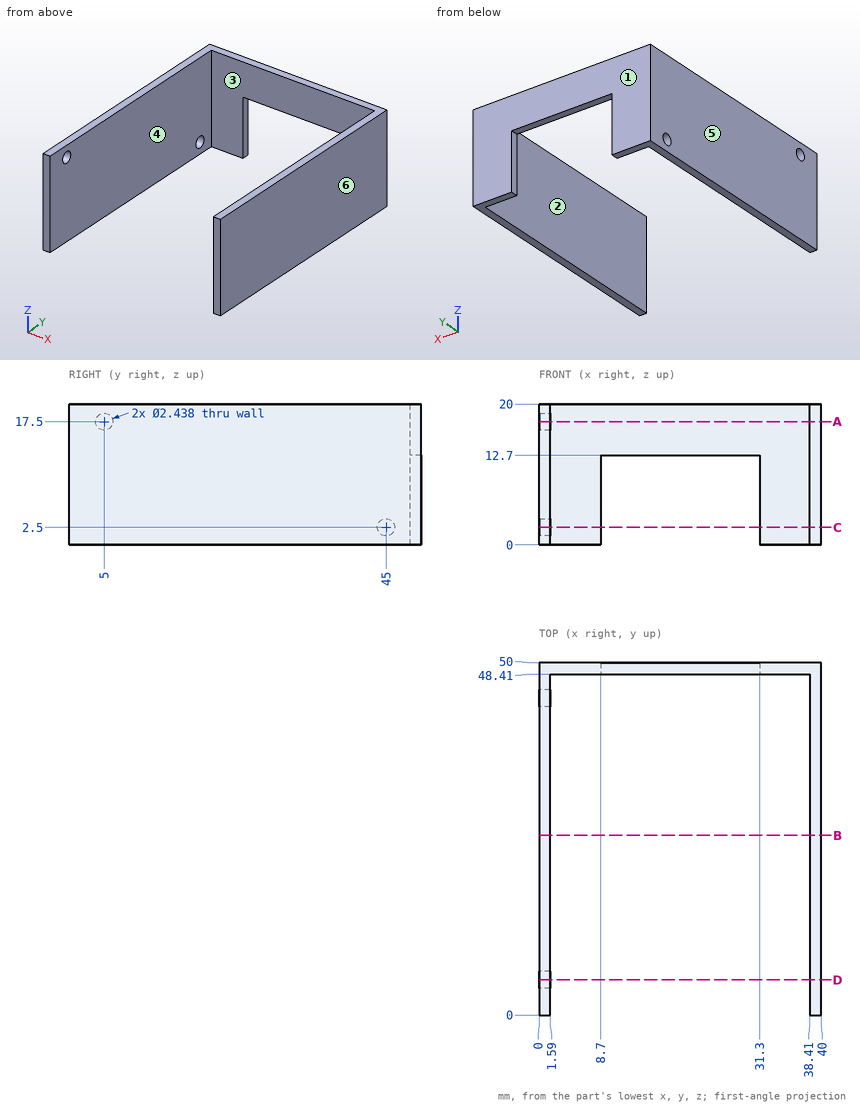
Geometry check sheet. Reference: drawing and pictorial views, mm from the part's lowest x, y, z. A direction names the side the tool comes from. Give positions to 0.01 mm unless a question says otherwise; leave off trailing zeros. Order: outer loops, then holes, each group sorted by start corner. A loop starts at its lowest first (then second) coordinate and runs counter-clockwise, first axis right, second up. Notation, with made-up numbers: M 65.5,9 L 85.5,9 A22 ccw 85.5,43 Z; hole C 11,20.5 d5. An arc over 180 degrees is marked long. Answer as a JSON object with one key per item and string values. Group by question number.
1) Cross-section at A-A (z = 17.5). Enter the section's corners in (x, y).
2) Scan lines: line 1 along X through (y, z) = (42.5, 4); line 2 along Y through (x, z) = (1.05, 17.5); line 3 along Y through (x, z) = (0.7, 2.5). Record each from-to range of solid material in increasing order. Write a range as [from, to].
3) Cross-section at D-D (y = 5). Enter the section's corners in (x, z).
4) Access from +Z, -Z, +X, -X, +Y, -Y to the whole of each face (thin tool, end or side, straight path). Record for the marked faces 1 and 2.
5) Mould release check, pull along X, two halves, no side actions. Record for the marked faces 3, 4, 5 and 6: released by +X, released by -X, zero draft, split by the parting line, or undercut.
6) Cross-section at B-B (y = 25.5). Enter the section's corners in (x, z).
7) Depth check by flat-ended pin: pin 1 Ø1.3 at (x, y) = (20.5, 49.5) entering from -Z; pin 2 Ø10 at (x, z) = (22.5, 17) entering from -Y. Enter the tip coordinate at first touch or a pass-through.
8) Cross-section at C-C (z = 2.5). Enter the section's corners in (x, y), then the cut area to 3 significant figures.
Result sheet:
{
 "1": {"outline": "M 0,0 L 1.59,0 L 1.59,3.78 L 0,3.78 Z; M 0,6.22 L 1.59,6.22 L 1.59,48.41 L 38.41,48.41 L 38.41,0 L 40,0 L 40,50 L 0,50 Z"},
 "2": {"line 1": "x = [0, 1.59], [38.41, 40]", "line 2": "y = [0, 3.78], [6.22, 50]", "line 3": "y = [0, 43.78], [46.22, 50]"},
 "3": {"outline": "M 0,0 L 1.59,0 L 1.59,16.28 L 0,16.28 Z; M 0,18.72 L 1.59,18.72 L 1.59,20 L 0,20 Z; M 38.41,0 L 40,0 L 40,20 L 38.41,20 Z"},
 "4": {"face 1": "+Z, -Z, +X, -X, +Y", "face 2": "+Z, -Z, -Y"},
 "5": {"face 3": "undercut", "face 4": "undercut", "face 5": "released by -X", "face 6": "released by +X"},
 "6": {"outline": "M 0,0 L 1.59,0 L 1.59,20 L 0,20 Z; M 38.41,0 L 40,0 L 40,20 L 38.41,20 Z"},
 "7": {"pin 1": "stops at z = 12.7", "pin 2": "stops at y = 48.41"},
 "8": {"outline": "M 0,0 L 1.59,0 L 1.59,43.78 L 0,43.78 Z; M 0,46.22 L 1.59,46.22 L 1.59,48.41 L 8.7,48.41 L 8.7,50 L 0,50 Z; M 31.3,48.41 L 38.41,48.41 L 38.41,0 L 40,0 L 40,50 L 31.3,50 Z", "area": "178 mm2"}
}
